CAD build for the part. Positions are in the model's coordinates, mm. A direction names the side the tool comes from. Coordinates: 2 decimals unless noted, no trailing zeros. Order: outer loops, then holes, each group sorted by start corner. A loop starts at its lowest first (then second) coordinate and runs counter-clockwise, first axis right, second up. Notation, with made-up numbers: M -31,-29 L -9,-29 A14 cw -9,-16 Z; hole C -12.5,-3 d6. An arc over 180 degrees is marked long. Write item = value, one per line.
from build123d import *

# Parameters (mm, degrees)
BOSS_EXTRUDE3_DEPTH = 5
BOSS_EXTRUDE4_DEPTH = 7.5


with BuildPart() as part:
    # Sketch1 → Boss-Extrude3 (new, symmetric)
    with BuildSketch(Plane.XY):
        with BuildLine():
            Line((-22, 110.563407366), (-22, 82.563407366))
            ThreePointArc((-22, 82.563407366), (0, 60.563407366), (22, 82.563407366))
            Line((22, 82.563407366), (22, 110.563407366))
            ThreePointArc((22, 110.563407366), (0, 132.563407366), (-22, 110.563407366))
        make_face()
        with BuildLine():
            ThreePointArc((-11, 96.563407366), (-11.707106781, 96.270514148), (-12, 95.563407366))
            Line((-12, 95.563407366), (-12, 82.563407366))
            ThreePointArc((-12, 82.563407366), (0, 70.563407366), (12, 82.563407366))
            Line((12, 82.563407366), (12, 95.563407366))
            ThreePointArc((12, 95.563407366), (11.707106781, 96.270514148), (11, 96.563407366))
            Line((11, 96.563407366), (10, 96.563407366))
            Line((10, 96.563407366), (10, 110.563407366))
            ThreePointArc((10, 110.563407366), (0, 120.563407366), (-10, 110.563407366))
            Line((-10, 110.563407366), (-10, 96.563407366))
            Line((-10, 96.563407366), (-11, 96.563407366))
        make_face(mode=Mode.SUBTRACT)
    extrude(amount=BOSS_EXTRUDE3_DEPTH, both=True)

    # Sketch1_5 → Boss-Extrude4 (add, symmetric)
    with BuildSketch(Plane.XY):
        with BuildLine():
            Line((28.804390709, 96.502814665), (22, 110.563407366))
            Line((22, 110.563407366), (22, 82.563407366))
            ThreePointArc((22, 82.563407366), (0, 60.563407366), (-22, 82.563407366))
            Line((-22, 82.563407366), (-22, 110.563407366))
            Line((-22, 110.563407366), (-28.804390709, 96.502814665))
            ThreePointArc((-28.804390709, 96.502814665), (-31.91369551, 80.214782471), (-26.453432284, 64.557410577))
            ThreePointArc((-26.453432284, 64.557410577), (-21.339698738, 45.404566029), (-29.2877286, 27.243879192))
            ThreePointArc((-29.2877286, 27.243879192), (0, -40), (29.2877286, 27.243879192))
            ThreePointArc((29.2877286, 27.243879192), (21.339698738, 45.404566029), (26.453432284, 64.557410577))
            ThreePointArc((26.453432284, 64.557410577), (31.91369551, 80.214782471), (28.804390709, 96.502814665))
        make_face()
        with BuildLine():
            Line((-11.878172589, -15.731008877), (-10, 10.563407366))
            ThreePointArc((-10, 10.563407366), (0, 20.563407366), (10, 10.563407366))
            Line((10, 10.563407366), (11.968538667, -16.568213586))
            ThreePointArc((11.968538667, -16.568213586), (0.434474391, -29.428724721), (-12, -17.436592634))
            ThreePointArc((-12, -17.436592634), (-11.969504398, -16.581628034), (-11.878172589, -15.731008877))
        make_face(mode=Mode.SUBTRACT)
    extrude(amount=BOSS_EXTRUDE4_DEPTH, both=True)


solid = part.part
(1) Slice it at C-C, the plane y = 0. Write the cut outline in (x, z).
Evaluation:
outline = M -40,-7.5 L -10.75,-7.5 L -10.75,7.5 L -40,7.5 Z; M 10.77,-7.5 L 40,-7.5 L 40,7.5 L 10.77,7.5 Z
(2) Slice it at D-D, the plane y = 67. Write the cut outline in (x, z), then the cut area to 3 significant figures.
Evaluation:
outline = M -27.96,-7.5 L -15.55,-7.5 L -15.55,-5 L 15.55,-5 L 15.55,-7.5 L 27.96,-7.5 L 27.96,7.5 L 15.55,7.5 L 15.55,5 L -15.55,5 L -15.55,7.5 L -27.96,7.5 Z
area = 683 mm²
(3) Slice it at A-A, the plane z = -2.75. Write the cut outline in (x, y), then the cut area to 3 significant figures.
Evaluation:
outline = M -29.29,27.24 A40 ccw long 29.29,27.24 A30 cw 26.45,64.56 A32 ccw 28.8,96.5 L 22,110.56 A22 ccw -22,110.56 L -28.8,96.5 A32 ccw -26.45,64.56 A30 cw Z; hole M -12,82.56 A12 ccw 12,82.56 L 12,95.56 A1 ccw 11,96.56 L 10,96.56 L 10,110.56 A10 ccw -10,110.56 L -10,96.56 L -11,96.56 A1 ccw -12,95.56 Z; hole M -11.88,-15.73 A12 ccw long 11.97,-16.57 L 10,10.56 A10 ccw -10,10.56 Z
area = 7,680 mm²
(4) Tool access for faces 1 (the face through (12, 89, 0)), 2 (the face through (-9, 20, -7.5)), 3 (the face through (0.48, 60.57, -6.23)), 4 (the face through (0.48, 132.56, 0.07)), 5 (the face through (14, 97, 5)): list every direction of +Z, -Z, +X, -X, +Y, -Y with a clear straight run to the whole face (end or side of a thin tool).
Evaluation:
face_1 = +Z, -Z
face_2 = -Z, +X, -X, +Y, -Y
face_3 = -Z, +Y
face_4 = +Z, -Z, +Y
face_5 = +Z, +Y
(5) Pin check, flat tips, straight feed: pin 1 Ø1 at (x, z) = (-22, -3) entering from -Y; pin 2 Ø4 at (y, z) = (113.5, -1) entering from +X; pin 3 Ø12 at (x, y) = (28, 49.5) entering from +Z; pin 4 Ø3 at (y, z) = (91.5, 6.5) entering from -X. Stop position of each tip, or through.
Evaluation:
pin_1 = -33.73
pin_2 = 21.98
pin_3 = through
pin_4 = -31.12
(6) Pull direction X, two halves, no side cores. Call faces 6 (the face through (-21.32, 45.69, 0.11)), 7 (the face through (-12, 89, 0)), 8 (the face through (-1.3, -39.98, 0.11)): +X half, -X half, draft (parallel to the pull), parting line (faces both ways), or undercut.
Evaluation:
face_6 = -X half
face_7 = undercut
face_8 = parting line
(7) Wall check: line 1 (X direction, y = 46.5, z = -3.25); line 2 (Y direction, x = -29, z = 1); line 3 (X direction, y = -21.5, z = 3.5). Give the ranges that are in metal, low to high. Write a range as from..to.
Evaluation:
line_1 = -21.28..21.28
line_2 = -27.55..27.56, 69.04..96.09
line_3 = -33.73..-11.29, 11.29..33.73
(8) Slice it at B-B, the plane x = 0. Write the cut outline in (y, z).
Evaluation:
outline = M -40,-7.5 L -29.44,-7.5 L -29.44,7.5 L -40,7.5 Z; M 20.56,-7.5 L 60.56,-7.5 L 60.56,-5 L 70.56,-5 L 70.56,5 L 60.56,5 L 60.56,7.5 L 20.56,7.5 Z; M 120.56,-5 L 132.56,-5 L 132.56,5 L 120.56,5 Z
